The listing builds one solid part. Answer for the finished solid, in the listing's coordinates (mm). Round coordinates to 2 decimals unless told otherwise and drop trailing zeros. Write each loop counter-clockwise with the first axis right and the second up, starting at its lowest first coordinate (ties: lowest second). Pieces come first, ordered by that corner, then holes.
Item 1: Find section B-B on x = 244. Give the vertices of the cut face in (y, z), then the cut area to 3 significant figures.
Item 2: Find section C-C on y = -39. Give the vertices of the cut face in (x, z).
Item 3: Find section A-A on z = 2.45. Give the number of separate pieces and of enclosed holes in the cut face, then the cut area to 3 significant figures.
Item 4: Each of these flat-tipped pins is pushed along its axis until it touches: pin 1 (1.5 mm diameter, centred on x = 99.5, y = 23, fed in from -Z); pin 2 (1.2 mm diameter, centred on y = 13, z = 2, fed in from -X); pin 3 (0.7 mm diameter, centred on y = 15.5, z = 2, fed in from -X); pin 4 (1 mm diameter, centred on y = 10, z = 2, fed in from -X). Where does it stop, or does it pass through?
Item 5: Find the intervals of material crossed by probe 1 along Y at (x, z) = (138, 1.3); probe 2 along Y at (x, z) = (70.5, 1.5); probe 3 along Y at (x, z) = (0, 2.55), in increasing order.
```python
from build123d import *

# Parameters (mm, degrees)
SKETCH1_R           = 1.5
SKETCH1_R_2         = 11
SKETCH1_R_3         = 1.55
SKETCH1_W           = 10
SKETCH1_H           = 4
BOSS_EXTRUDE1_DEPTH = 4
FILLET1_R           = 8


with BuildPart() as part:
    # Sketch1 → Boss-Extrude1 (new body)
    with BuildSketch(Plane.XY):
        with BuildLine():
            Line((-12, 34), (-26, 3.5))
            Line((-26, 3.5), (-26, -20))
            Line((-26, -20), (-12, -65))
            Line((-12, -65), (18, -65))
            Line((18, -65), (18, -45))
            Line((18, -45), (18, -6.1))
            Line((18, -6.1), (306.5, -6.1))
            Line((306.5, -6.1), (306.5, -17))
            Line((306.5, -17), (325, -17))
            Line((325, -17), (325, -3))
            Line((325, -3), (315, -3))
            ThreePointArc((315, -3), (312, 0), (315, 3))
            Line((315, 3), (325, 3))
            Line((325, 3), (325, 6))
            Line((325, 6), (327, 6))
            Line((327, 6), (327, 15))
            ThreePointArc((327, 15), (321.435028843, 28.435028843), (308, 34))
            Line((308, 34), (-12, 34))
        make_face()
        with Locations((21.920310217, 0)):
            Circle(SKETCH1_R, mode=Mode.SUBTRACT)
        with Locations((0, -21.920310217)):
            Circle(SKETCH1_R, mode=Mode.SUBTRACT)
        with Locations((-21.920310217, 0)):
            Circle(SKETCH1_R, mode=Mode.SUBTRACT)
        Circle(SKETCH1_R_2, mode=Mode.SUBTRACT)
        with Locations((-9.05, 26.5)):
            Circle(SKETCH1_R_3, mode=Mode.SUBTRACT)
        with Locations((15.05, 18.5)):
            Circle(SKETCH1_R_3, mode=Mode.SUBTRACT)
        with Locations((-9.05, -49.5)):
            Circle(SKETCH1_R_3, mode=Mode.SUBTRACT)
        with Locations((15.05, -57.5)):
            Circle(SKETCH1_R_3, mode=Mode.SUBTRACT)
        with Locations((70.5, 6.5)):
            Circle(SKETCH1_R_3, mode=Mode.SUBTRACT)
        with Locations((70.5, 19.5)):
            Circle(SKETCH1_R_3, mode=Mode.SUBTRACT)
        with Locations((17, 13)):
            Rectangle(SKETCH1_W, SKETCH1_H, mode=Mode.SUBTRACT)
        with Locations((142, 13)):
            Rectangle(SKETCH1_W, SKETCH1_H, mode=Mode.SUBTRACT)
        with Locations((302, 13)):
            Rectangle(SKETCH1_W, SKETCH1_H, mode=Mode.SUBTRACT)
        Polygon((53.5, 11), (58.5, 11), (58.5, 9.95), (61.5, 9.95), (61.5, 7.5), (66.5, 7.5), (66.5, 11), (71, 11), (71, 9.5), (71.5, 9.5), (71.5, 9.7), (74, 9.7), (74, 11), (78.5, 11), (78.5, 15), (74, 15), (74, 16.3), (71.5, 16.3), (71.5, 16.5), (71, 16.5), (71, 15), (66.5, 15), (66.5, 18.5), (61.5, 18.5), (61.5, 16.05), (58.5, 16.05), (58.5, 15), (53.5, 15), align=None, mode=Mode.SUBTRACT)
    extrude(amount=BOSS_EXTRUDE1_DEPTH)

    # Fillet1
    fillet1_edges = [part.edges().sort_by_distance(p)[0] for p in [
        (18, -6.1, 2),
    ]]
    fillet(fillet1_edges, radius=FILLET1_R)


solid = part.part
```
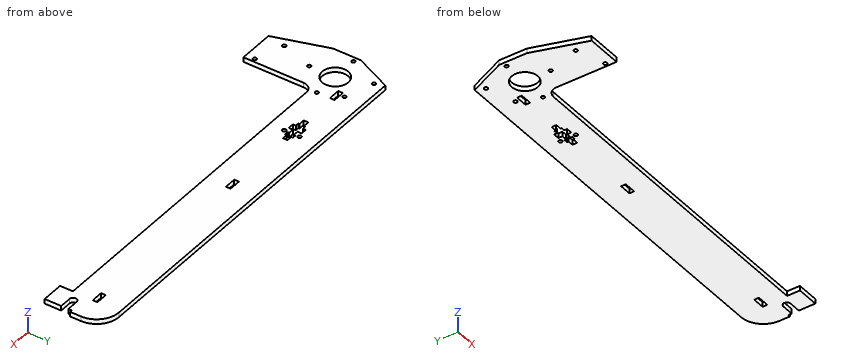
Check values:
1. outline: (-6.1, 0) - (34, 0) - (34, 4) - (-6.1, 4) - close
1. area: 160 mm2
2. outline: (-20.09, 0) - (18, 0) - (18, 4) - (-20.09, 4) - close
3. separate pieces: 1
3. enclosed holes: 14
3. area: 15,500 mm2
4. pin 1: stops at z = 0
4. pin 2: stops at x = -21.91
4. pin 3: stops at x = -20.65
4. pin 4: stops at x = -23.25
5. probe 1: y = -6.1 to 11, 15 to 34
5. probe 2: y = -6.1 to 4.95, 8.05 to 11, 15 to 17.95, 21.05 to 34
5. probe 3: y = -65 to -23.42, -20.42 to -11, 11 to 34
